The listing builds one solid part. Answer for the finished solid, in the listing's coordinates (mm). Coordinates: 2 decimals unless noted, no trailing zeros. Order: outer loops, then holes, each group sorted by start corner. A loop starts at its lowest first (then second) coordinate and runs counter-clockwise, first axis right, second up. Notation, with made-up numbers: (-23, 59.25) - (32, 59.25) arc R17 ccw to (32, 69.25) - close; hole circle Ø1 at (6.25, 82.5). An arc over 180 degrees is marked (long way). Use a Markdown table: item, result. Add a question column.
Item 1: Find the intervals of material crossed by line 1 along X through (y, z) = (4.5, -4); line 2 along Z through (x, y) = (7.5, 4.25); line 3 along Z through (x, y) = (1.25, 3.5), in increasing order.
Item 2: The part is cut by section D-D, the plane y = 5.25. State how many separate pieces and enclosed holes the cut face has, then the cut area to 3 significant figures.
Item 3: The mould has two halves that part along X. Classify faces 1 (the cylindrical face through (-6.58, 3.13, -2.31)), 2 (the cylindrical face through (-7.7, 3.1, -10.1)), 3 (the flat face through (-3, 0, 3)): released by +X, released by -X, zero draft, split by the parting line, or undercut.
Item 4: The part is cut by section C-C, the plane z = -2.75. Give the vertices of the cut face in (x, y).
Item 5: The part is cut by section A-A, the plane z = 0. Give the vertices of the cut face in (x, y).
Item 6: A flat-ended cylindrical pin translates along its axis: P1, Ø6, axis at x = 0, z = 0, coming from the +Y side. Find the tip coordinate at first contact, or state that the pin passes through.
Item 7: The part is cut by section B-B, the plane x = 0. Give the vertices of the cut face in (y, z).
from build123d import *

# Parameters (mm, degrees)
SKETCH1_R   = 12.7
SKETCH1_R_2 = 1.905
SKETCH1_R_3 = 3.2385
BASE_DEPTH  = 6.35


with BuildPart() as part:
    # Sketch1 → base (new body)
    with BuildSketch(Plane(origin=(0, 0, 0), x_dir=(1, 0, 0), z_dir=(0, 1, 0))):
        with Locations(Location((0, 0, 0), (0, 0, 270))):
            Circle(SKETCH1_R)
        with Locations(Location((0, 8.255, 0), (0, 0, 270))):
            Circle(SKETCH1_R_2, mode=Mode.SUBTRACT)
        with Locations(Location((0, 0, 0), (0, 0, 270))):
            Circle(SKETCH1_R_3, mode=Mode.SUBTRACT)
        with Locations(Location((7.149039708, 4.1275, 0), (0, 0, 270))):
            Circle(SKETCH1_R_2, mode=Mode.SUBTRACT)
        with Locations(Location((7.149039708, -4.1275, 0), (0, 0, 270))):
            Circle(SKETCH1_R_2, mode=Mode.SUBTRACT)
        with Locations(Location((0, -8.255, 0), (0, 0, 270))):
            Circle(SKETCH1_R_2, mode=Mode.SUBTRACT)
        with Locations(Location((-7.149039708, -4.1275, 0), (0, 0, 270))):
            Circle(SKETCH1_R_2, mode=Mode.SUBTRACT)
        with Locations(Location((-7.149039708, 4.1275, 0), (0, 0, 270))):
            Circle(SKETCH1_R_2, mode=Mode.SUBTRACT)
    extrude(amount=BASE_DEPTH)


solid = part.part
Solution:
| question | item | result |
|---|---|---|
| 1 | line 1 | x = -12.05 to -9.05, -5.25 to 5.25, 9.05 to 12.05 |
| 1 | line 2 | z = -10.25 to -6, -2.26 to 2.26, 6 to 10.25 |
| 1 | line 3 | z = -12.64 to -9.69, -6.82 to -2.99, 2.99 to 6.82, 9.69 to 12.64 |
| 2 | separate pieces | 1 |
| 2 | enclosed holes | 7 |
| 2 | area | 405 mm2 |
| 3 | face 1 | undercut |
| 3 | face 2 | split by the parting line |
| 3 | face 3 | zero draft |
| 4 | outline | (-12.4, 0) - (-8.46, 0) - (-8.46, 6.35) - (-12.4, 6.35) - close; (-5.83, 0) - (-1.71, 0) - (-1.71, 6.35) - (-5.83, 6.35) - close; (1.71, 0) - (5.83, 0) - (5.83, 6.35) - (1.71, 6.35) - close; (8.46, 0) - (12.4, 0) - (12.4, 6.35) - (8.46, 6.35) - close |
| 5 | outline | (-12.7, 0) - (-3.24, 0) - (-3.24, 6.35) - (-12.7, 6.35) - close; (3.24, 0) - (12.7, 0) - (12.7, 6.35) - (3.24, 6.35) - close |
| 6 | P1 | passes through |
| 7 | outline | (0, -12.7) - (6.35, -12.7) - (6.35, -10.16) - (0, -10.16) - close; (0, -6.35) - (6.35, -6.35) - (6.35, -3.24) - (0, -3.24) - close; (0, 3.24) - (6.35, 3.24) - (6.35, 6.35) - (0, 6.35) - close; (0, 10.16) - (6.35, 10.16) - (6.35, 12.7) - (0, 12.7) - close |
